Source: CAD feature listing. Evaluate the final solid. Frame: model axes, mm. Coordinates: 2 decimals unless noted, no trailing zeros. Order: outer loops, then holes, each group sorted by start corner. A loop starts at its lowest first (then second) coordinate and runs counter-clockwise, first axis right, second up.
Item 1: Ray query, line 1 (X direction, y = -396.5, z = 2.05); line 2 (Y direction, x = -165, z = 1.35); line 3 (X direction, y = 378.5, z = 3.55). Return the intervals inside material, ascending.
Item 2: Section B-B on y = -254. Return the cut outline in (x, z), then the cut area to 4 significant figures.
Item 3: Contact query for flat-ended pins moving along their axis: P1, Ø2.5, axis at x = -130, z = 3, coming from the -Y side; P2, Ø4.5, axis at x = 100, y = 378.5, coming from the -Z side; P3, Ø2.5, axis at y = -122, z = 3, coming from the -X side. Output: stop coordinate, or through.
Item 4: Section A-A on z = 1.05. Return the cut outline in (x, y), then the cut area to 3 significant figures.
Item 5: Section C-C on x = -145. Return the cut outline in (y, z).
from build123d import *

# Parameters (mm, degrees)
PAD_DEPTH    = 5
SKETCH001_R  = 2
POCKET_DEPTH = 5


with BuildPart() as part:
    # Sketch → Pad (new body)
    with BuildSketch(Plane.XY):
        Polygon((-107.5, 438.5), (107.5, 438.5), (107.5, -456.5), (-107.5, -456.5), (-107.5, -7.5), (-172.5, -7.5), (-172.5, 438.5), align=None)
    extrude(amount=PAD_DEPTH)

    # Sketch001 → Pocket (cut)
    with BuildSketch(Plane.XY.offset(5)):
        with Locations((-165, 378.5)):
            Circle(SKETCH001_R)
        with Locations((-165, 52.5)):
            Circle(SKETCH001_R)
        with Locations((-100, -396.5)):
            Circle(SKETCH001_R)
        with Locations((100, -396.5)):
            Circle(SKETCH001_R)
        with Locations((100, 378.5)):
            Circle(SKETCH001_R)
    extrude(amount=-POCKET_DEPTH, mode=Mode.SUBTRACT)


solid = part.part
Answer list:
1. line 1: x = -107.5 to -102, -98 to 98, 102 to 107.5
1. line 2: y = -7.5 to 50.5, 54.5 to 376.5, 380.5 to 438.5
1. line 3: x = -172.5 to -167, -163 to 98, 102 to 107.5
2. outline: (-107.5, 0) - (107.5, 0) - (107.5, 5) - (-107.5, 5) - close
2. area: 1,075 mm2
3. P1: stops at y = -7.5
3. P2: stops at z = 0
3. P3: stops at x = -107.5
4. outline: (-172.5, -7.5) - (-107.5, -7.5) - (-107.5, -456.5) - (107.5, -456.5) - (107.5, 438.5) - (-172.5, 438.5) - close; hole circle Ø4 at (-165, 52.5); hole circle Ø4 at (-165, 378.5); hole circle Ø4 at (-100, -396.5); hole circle Ø4 at (100, -396.5); hole circle Ø4 at (100, 378.5)
4. area: 221,000 mm2
5. outline: (-7.5, 0) - (438.5, 0) - (438.5, 5) - (-7.5, 5) - close
